Can you work these out from the model? Positions are in its coordinate system, mm. A direction names the side the tool comes from. Coordinates: 2 decimals unless noted, no trailing zeros. Loops run counter-clockwise (first coordinate to the right, second up) from the corner with the lowest first, then second, coordinate; pieces in that order, holes last.
```python
from build123d import *

# Parameters (mm, degrees)
FILLET_1_R          = 0.7
FILLET_4_R          = 0.8
CUT_EXTRUDE_START   = -0.1
CUT_EXTRUDE_3_DEPTH = 0.1


# Read off the part's stored shape, not the designer's step: Вырез-Вытянуть-Тонкостенный3
with BuildPart() as part:
    # Эскиз2 → Повернуть1 (revolve)
    with BuildSketch(Plane.XY):
        with BuildLine():
            Line((0, 0), (0, 4.85))
            Line((0, 4.85), (-0.1, 4.85))
            Line((-0.1, 4.85), (-0.1, 6.4))
            Line((-0.1, 6.4), (21.2, 6.4))
            ThreePointArc((21.2, 6.4), (22.45, 5.7), (23.7, 6.4))
            Line((23.7, 6.4), (25.7, 6.4))
            Line((25.7, 6.4), (25.7, 4.15))
            Line((25.7, 4.15), (25.1, 4.15))
            Line((25.1, 4.15), (25.1, 3.75))
            Line((25.1, 3.75), (25.7, 3.75))
            Line((25.7, 3.75), (25.7, 0))
            Line((25.7, 0), (0, 0))
        make_face()
    revolve(axis=Axis((25.7, 0, 0), (-1, 0, 0)))

    # Скругление1
    fillet_1_edges = [part.edges().sort_by_distance(p)[0] for p in [
        (25.7, -6.4, 0),
        (-0.1, -6.4, 0),
    ]]
    fillet(fillet_1_edges, radius=FILLET_1_R)

    # Скругление4
    fillet_4_edges = [part.edges().sort_by_distance(p)[0] for p in [
        (21.2, -6.4, 0),
        (23.7, -6.4, 0),
    ]]
    fillet(fillet_4_edges, radius=FILLET_4_R)

    # Вырез-Вытянуть-Тонкостенный3 outline → Вырез-Вытянуть-Тонкостенный3 (cut)
    with BuildSketch(Plane.ZY.offset(CUT_EXTRUDE_START)):
        Polygon((-3.872114317, -2.29330127), (0, -0.057735027), (3.872114317, -2.29330127), (3.922114317, -2.20669873), (0.05, 0.028867513), (0.05, 4.5), (-0.05, 4.5), (-0.05, 0.028867513), (-3.922114317, -2.20669873), align=None)
    extrude(amount=CUT_EXTRUDE_3_DEPTH, mode=Mode.SUBTRACT)


solid = part.part
```
Item 1: Suppose I cut it at B-B, the plane x = 22.5. Please give me the cut outline in (y, z).
Results are:
outline: circle Ø11.4 at (0, 0)
Item 2: On a 3-axis mill with a long thin cutter (end or side, diameter ignored), from which of +Z, -Z, +X, -X, +Y, -Y can I reach the whole of each face in a straight line? I mean faces 1 (the face through (-0.1, 3, -4)), 2 (the face through (25.404, -3.746, -0.165)), 3 (the face through (0, -1, 0)). Say none if no direction works.
Results are:
face 1: +Z, -Z, -X, +Y, -Y
face 2: +X
face 3: -X
Item 3: Suppose I cut it at A-A, the plane x = 6.75. Please give me the cut outline in (y, z), plus the area to 3 significant figures.
Results are:
outline: circle Ø12.8 at (0, 0)
area: 129 mm2
Item 4: I'm going to push flat-ended pins straight in: P1, Ø2, axis at y = 1.5, z = 1.5, coming from the -X side; P2, Ø1, axis at x = 16, y = -2.5, coming from the -Z side; P3, Ø6, axis at x = 15.5, z = -5, coming from the +Y side. Where does each tip first touch, or does it pass through?
Results are:
P1: stops at x = 0
P2: stops at z = -6.08
P3: stops at y = 6.08
Item 5: I need wall thicknesses on line 1 along Y through (x, z) = (25.4, 0); line 2 along Y through (x, z) = (25.5, 0); line 3 along Z through (x, y) = (25.55, 0). Which ranges of each line are inside material? Lowest first, please.
Results are:
line 1: y = -6.27 to -4.15, -3.75 to 3.75, 4.15 to 6.27
line 2: y = -6.19 to -4.15, -3.75 to 3.75, 4.15 to 6.19
line 3: z = -6.13 to -4.15, -3.75 to 3.75, 4.15 to 6.13
